Geometry: final body of the model. Coordinates: model frame, mm. A direction names the side the tool comes from. Give positions to 0.01 mm unless a question says otherwise; leave off trailing zeros. Loops run counter-clockwise (first coordinate to the right, second up) from the corner with the lowest first, then second, coordinate; pieces in that order, holes last.
from build123d import *

# Parameters (mm, degrees)
SKETCH1_R            = 2.1
BOSS_EXTRUDE2_DEPTH  = 200
CUT_EXTRUDE1_DEPTH   = 201
FILLET1_R            = 0.25
FILLET1_OF_MIRROR1_R = 0.25


with BuildPart() as part:
    # Sketch1 → Boss-Extrude2 (new body)
    with BuildSketch(Plane.XY):
        Polygon((8.199993721, -10), (9.999993721, -10), (9.999993721, -4.63999575), (8.199993721, -2.84), (8.199993721, -5.800653822), (6.861313026, -5.800653822), (3.900652213, -2.84), (3.900652213, 2.84), (6.559993721, 5.499347787), (8.199993721, 5.499347787), (8.199993721, 2.84), (9.999993721, 4.64000425), (9.999993721, 10), (4.63999575, 10), (2.84, 8.2), (5.499325592, 8.2), (5.499325592, 6.56), (2.84, 3.900668129), (-2.84, 3.900668129), (-5.49933815, 6.56), (-5.49933815, 8.2), (-2.84, 8.2), (-4.64000425, 10), (-10.000006279, 10), (-10.000006279, 4.63999575), (-8.200006279, 2.84), (-8.200006279, 5.499347787), (-6.560006279, 5.499347787), (-3.900652213, 2.84), (-3.900652213, -2.84), (-6.861299044, -5.800653822), (-8.200006279, -5.800653822), (-8.200006279, -2.84), (-10.000006279, -4.64000425), (-10.000006279, -10), (-8.200006279, -10), (-8.200006279, -7.300653822), (-6.239977665, -7.300653822), (-2.84, -3.900668129), (2.84, -3.900668129), (6.239993721, -7.300653822), (8.199993721, -7.300653822), align=None)
        Circle(SKETCH1_R, mode=Mode.SUBTRACT)
    boss_extrude2 = extrude(amount=BOSS_EXTRUDE2_DEPTH)

    # Sketch2 → Cut-Extrude1 (cut, through all)
    with BuildSketch(Plane.XY.offset(200)):
        Polygon((-8.200006279, 6.569347787), (-8.200006279, 8.2), (-6.56933815, 8.2), (-6.56933815, 7.630009211), (-7.62999707, 6.569347787), align=None)
        Polygon((8.199993721, 8.2), (8.199993721, 6.569347787), (7.629987016, 6.569347787), (6.569325592, 7.630006706), (6.569325592, 8.2), align=None)
    cut_extrude1 = extrude(amount=-CUT_EXTRUDE1_DEPTH, mode=Mode.SUBTRACT)

    # Fillet1
    fillet1_edges = [part.edges().sort_by_distance(p)[0] for p in [
        (9.999993721, -4.63999575, 100),
        (-10.000006279, -4.64000425, 100),
        (-8.200006279, -2.84, 100),
        (-8.200006279, 2.84, 100),
        (-10.000006279, 4.63999575, 100),
        (-10.000006279, 10, 100),
        (-4.64000425, 10, 100),
        (-2.84, 8.2, 100),
        (2.84, 8.2, 100),
        (4.63999575, 10, 100),
        (9.999993721, 10, 100),
        (9.999993721, 4.64000425, 100),
        (8.199993721, 2.84, 100),
        (8.199993721, -2.84, 100),
    ]]
    fillet(fillet1_edges, radius=FILLET1_R)

    # Mirror1: Boss-Extrude2 across plane
    add(boss_extrude2.mirror(Plane(origin=(0, -10, 0), x_dir=(0, 0, 1), z_dir=(0, -1, 0))))

    # Fillet1 of Mirror1
    fillet1_of_mirror1_edges = [part.edges().sort_by_distance(p)[0] for p in [
        (9.999993721, -15.36000425, 100),
        (-10.000006279, -15.35999575, 100),
        (-8.200006279, -17.16, 100),
        (-8.200006279, -22.84, 100),
        (-10.000006279, -24.63999575, 100),
        (-10.000006279, -30, 100),
        (-4.64000425, -30, 100),
        (-2.84, -28.2, 100),
        (2.84, -28.2, 100),
        (4.63999575, -30, 100),
        (9.999993721, -30, 100),
        (9.999993721, -24.64000425, 100),
        (8.199993721, -22.84, 100),
        (8.199993721, -17.16, 100),
    ]]
    fillet(fillet1_of_mirror1_edges, radius=FILLET1_OF_MIRROR1_R)

    # Mirror2: Cut-Extrude1 across plane
    add(cut_extrude1.mirror(Plane(origin=(0, -10, 0), x_dir=(0, 0, 1), z_dir=(0, -1, 0))), mode=Mode.SUBTRACT)


solid = part.part
Item 1: Section query A-A on x = 0. Return loops of the section in (y, z).
Values follow:
outline: (-23.9, 0) - (-22.1, 0) - (-22.1, 200) - (-23.9, 200) - close; (-17.9, 0) - (-16.1, 0) - (-16.1, 200) - (-17.9, 200) - close; (-3.9, 0) - (-2.1, 0) - (-2.1, 200) - (-3.9, 200) - close; (2.1, 0) - (3.9, 0) - (3.9, 200) - (2.1, 200) - close
Item 2: Ray query, probe 1 along Y at (x, z) = (0, 158.5); probe 2 along Y at (x, z) = (-8, 60); probe 3 along X at (y, z) = (-5.5, 127). Return the intervals inside material, ascending.
Values follow:
probe 1: y = -23.9 to -22.1, -17.9 to -16.1, -3.9 to -2.1, 2.1 to 3.9
probe 2: y = -30 to -28.2, -26.57 to -25.5, -14.2 to -12.7, -7.3 to -5.8, 5.5 to 6.57, 8.2 to 10
probe 3: x = -10 to -8.2, -6.56 to -4.44, 4.44 to 6.56, 8.2 to 10
Item 3: Draft query along Y for faces 1 (the face through (0, 3.901, 99)), 2 (the face through (-10, 7, 99)), 3 (the face through (0, -16.099, 99)). Return one class per face: +Y half, -Y half, draft (parallel to the pull), parting line (faces both ways), or undercut.
Values follow:
face 1: +Y half
face 2: draft
face 3: undercut
Item 4: Section query B-B on y = -20. Return loops of the section in (x, z).
Values follow:
outline: (-3.9, 0) - (-2.1, 0) - (-2.1, 200) - (-3.9, 200) - close; (2.1, 0) - (3.9, 0) - (3.9, 200) - (2.1, 200) - close
Item 5: Section query C-C on z = 129.5. Give the number of separate pieces and of enclosed holes in the cut face, plus the area to 3 significant figures.
Values follow:
separate pieces: 1
enclosed holes: 7
area: 289 mm2
Item 6: Pin query (flat end, axial travel): pin 1 (4 mm diameter, centred on x = 1, y = -5, fed in from -Z); pin 2 (4 mm diameter, centred on y = 0, z = 48, fed in from +X); pin 3 (5 mm diameter, centred on x = -0.5, z = 169.5, fed in from +Y); pin 4 (1 mm diameter, centred on x = 4, z = 145.5, fed in from -Y). Return the tip coordinate at first contact, or that it passes through.
Values follow:
pin 1: stops at z = 0
pin 2: stops at x = 3.9
pin 3: stops at y = 4.06
pin 4: stops at y = -29.86
Item 7: Set-up query: faces 4 (the face through (0, -23.901, 99)), 5 (the face through (-3.901, -20, 99)), 6 (the face through (-4.56, -14.38, 98.6)), 7 (the face through (3.901, 0, 99)). Return all of +Z, -Z, +X, -X, +Y, -Y with unobstructed straight access to the full face (end or side cutting, diameter ignored); none if empty.
Values follow:
face 4: +Z, -Z, -Y
face 5: +Z, -Z, -X
face 6: +Z, -Z
face 7: +Z, -Z, +X
